Can you work these out from the model? Positions are in its coordinate system, mm. A direction names the side the tool comes from. Round coordinates to 2 decimals unless told otherwise and drop trailing zeros. Order: outer loops, then holes, each group sorted by start corner. A loop starts at its lowest first (then second) coordinate and runs counter-clockwise, first axis right, second up.
Q1. If we section it at C-C (z = 28.5): Please give me the cut outline in (x, y).
Q2. We'd pull the mould along Y, two halves only. Please class faces 3 (the face through (-1.63, 9.762, 15.219)), 4 (the face through (-5.966, 29.287, 21.339)), 5 (the face through (4, 10, 17.754)), 6 (the face through (1, 12, 12.754)): pulls with the +Y half, pulls with the -Y half, needs draft (parallel to the pull), parting line crosses it, or undercut.
Q3. Will these pins go through, and if not, where does the flat tip stop? P1, Ø10, axis at y = 18.5, z = 16.5, coming from the +X side; P2, Ø9, axis at x = 3, y = -5, coming from the +Z side; P3, Ø8, axis at x = 23.5, z = 19.5, coming from the -Y side; P4, Ø18, axis at x = 0.54, y = 0, coming from the -Z side (1 decimal).
Q4. If I drill on line 1 (X direction, y = 0, z = 21.5); line 2 (X direction, y = 0, z = 15.2); line 3 (Y direction, x = 9.5, z = 15.5), over which ranges is the centre line in solid material (lowest first)?
Q5. If we section it at A-A (y = 0): Please give me the cut outline in (x, z), plus the area to 3 significant figures.
Q6. For faces 1 (the face through (12, -13, 29.754)), 2 (the face through (-2.714, 14.643, 22.684)), which set-ups out of +Z, -Z, +X, -X, +Y, -Y let a thin tool reach every point of the face, with its end or its side?
Q7. If we section it at B-B (z = 23.75): Please give me the cut outline in (x, y), plus the area to 3 significant figures.
from build123d import *

# Parameters (mm, degrees)
F2_R    = 2.3981299458
F3_SIZE = 2


with BuildPart() as f1:
    # F0 (on Front) → F1 (revolve)
    with BuildSketch(Plane.XZ):
        Polygon((15.5377323945, 17.7536051821), (10.5377323945, 17.7536051821), (10.5377323945, 12.7536051821), (30.5377323945, 12.7536051821), (30.5377323945, 29.7536051821), (15.5377323945, 29.7536051821), align=None)
    revolve(axis=Axis((0.5377323945, 0, 22.511664778), (0, 0, -1)))

    # F2
    f2_edges = [f1.edges().sort_by_distance(p)[0] for p in [
        (-29.462268, 0, 29.753605),
        (-29.462268, 0, 12.753605),
    ]]
    fillet(f2_edges, radius=F2_R)

    # F3
    f3_edges = [f1.edges().sort_by_distance(p)[0] for p in [
        (-14.462268, 0, 29.753605),
    ]]
    chamfer(f3_edges, length=F3_SIZE)


solid = f1.part
Solution:
1. outline: circle Ø59.42 at (0.54, 0); hole circle Ø31.49 at (0.54, 0)
2. face 3: undercut
2. face 4: parting line crosses it
2. face 5: undercut
2. face 6: needs draft
3. P1: stops at x = 27.33
3. P2: stops at z = 17.75
3. P3: stops at y = -23.25
3. P4: passes through
4. line 1: x = -29.46 to -14.46, 15.54 to 30.54
4. line 2: x = -29.46 to -9.46, 10.54 to 30.54
4. line 3: y = -28.63 to -4.44, 4.44 to 28.63
5. outline: (-29.46, 15.15) arc R2.4 ccw to (-27.06, 12.75) - (-9.46, 12.75) - (-9.46, 17.75) - (-14.46, 17.75) - (-14.46, 27.75) - (-16.46, 29.75) - (-27.06, 29.75) arc R2.4 ccw to (-29.46, 27.36) - close; (10.54, 12.75) - (28.14, 12.75) arc R2.4 ccw to (30.54, 15.15) - (30.54, 27.36) arc R2.4 ccw to (28.14, 29.75) - (17.54, 29.75) - (15.54, 27.75) - (15.54, 17.75) - (10.54, 17.75) - close
5. area: 551 mm2
6. face 1: +Z, +X, -X, +Y, -Y
6. face 2: +Z
7. outline: circle Ø60 at (0.54, 0); hole circle Ø30 at (0.54, 0)
7. area: 2,120 mm2
